```python
from build123d import *

# Parameters (mm, degrees)
SKETCH1_W                                           = 57.650718963
SKETCH1_H                                           = 45.709483456
BOSS_EXTRUDE1_DEPTH                                 = 5
CSK_FOR_M3_COUNTERSUNK_FLAT_HEAD_SCREW2_D           = 3.4
CSK_FOR_M3_COUNTERSUNK_FLAT_HEAD_SCREW2_CSINK_D     = 6.3
CSK_FOR_M3_COUNTERSUNK_FLAT_HEAD_SCREW2_CSINK_ANGLE = 90


with BuildPart() as part:
    # Sketch1 → Boss-Extrude1 (new body)
    with BuildSketch(Plane.XY):
        with Locations((-28.825359482, -22.854741728)):
            Rectangle(SKETCH1_W, SKETCH1_H)
    extrude(amount=BOSS_EXTRUDE1_DEPTH)

    # CSK for M3 Countersunk Flat Head Screw2 (through all)
    with Locations(Plane.XY.offset(5)):
        with Locations((-36.815052067, -20.667361914)):
            CounterSinkHole(CSK_FOR_M3_COUNTERSUNK_FLAT_HEAD_SCREW2_D / 2, CSK_FOR_M3_COUNTERSUNK_FLAT_HEAD_SCREW2_CSINK_D / 2, counter_sink_angle=CSK_FOR_M3_COUNTERSUNK_FLAT_HEAD_SCREW2_CSINK_ANGLE)

    # Sketch13 → CSK for M5 Countersunk Flat Head Screw1 (revolve, cut)
    with BuildSketch(Plane(origin=(-14.434702808, -26.976225799, 0), x_dir=(0, 1, 0), z_dir=(1, 0, 0))):
        Polygon((0, 0), (0, 5), (2.75, 5), (2.75, 2.45), (5.2, 0), align=None)
    revolve(axis=Axis((-14.434702808, -26.976225799, -6.35), (0, 0, 1)), mode=Mode.SUBTRACT)


solid = part.part
```
Geometry: final body of the model. Coordinates: model frame, mm. Round coordinates to 2 decimals unless told otherwise and drop trailing zeros. Write each loop counter-clockwise with the first axis right and the second up, starting at its lowest first coordinate (ties: lowest second). Pieces come first, ordered by that corner, then holes. Notation, with made-up numbers: M 66,0.5 L 71,0.5 A24 ccw 71,36.5 Z; hole C 16.25,-22 d5. An arc over 180 degrees is marked long. Answer in a Markdown table with one row per item. Add a question column.
(1) Cut plane A-A, the plane z = 1.45. Return the cut outline in (x, y).
(2) Draft query along X for faces 1 (the face through (-29, -45.709, 2)), 2 (the face through (-57.651, -23, 2)), 3 (the face through (-17.16, -27.33, 3.71)), 4 (the face through (0, -23, 2)). Return one class per face: pulls with the +X half, pulls with the -X half, needs draft (parallel to the pull), parting line crosses it, or undercut.
(3) Contact query for flat-ended pins moving along their axis: pin 1 (7 mm diameter, centred on x = -14.43, y = -26.98, fed in from +Z); pin 2 (4.5 mm diameter, centred on x = -36.82, y = -20.67, fed in from +Z). Output: stop coordinate, or through.
(4) Ray query, L1, parallel to X at y = -27, z = 0.8; L2, parallel to Y at x = -11, z = 1.15; L3, parallel to X at y = -22, z = 1. Return the intervals inside material, ascending.
Established:
| question | item | result |
|---|---|---|
| 1 | outline | M -57.65,-45.71 L 0,-45.71 L 0,0 L -57.65,0 Z; hole C -36.82,-20.67 d3.4; hole C -14.43,-26.98 d7.5 |
| 2 | face 1 | needs draft |
| 2 | face 2 | pulls with the -X half |
| 2 | face 3 | undercut |
| 2 | face 4 | pulls with the +X half |
| 3 | pin 1 | z = 5 |
| 3 | pin 2 | z = 4.11 |
| 4 | L1 | -57.65 to -18.83, -10.03 to 0 |
| 4 | L2 | -45.71 to -29.12, -24.83 to 0 |
| 4 | L3 | -57.65 to -37.87, -35.76 to 0 |
